Solid Edge part; units mm, degrees
sketch "Sketch1" plane through (0, 0, 0) normal (0, -1, 0) x (1, 0, 0)
  line L0 (12, 0) -> (12, 0.95)
  line L1 (12, 0.95) -> (1.25, 0.95)
  line L2 (1.25, 1.63) -> (1.25, 0.95)
  spline S0 degree 3 poles (0, 0) (0, 0.7831) (0.4356, 1.448) (1.25, 1.63) knots 0 0 0 0 1 1 1 1
revolve "RevolvedProtrusion1" add sketch "Sketch1" angle 360 about axis through (0, 0, 0) along (1, 0, 0)
sketch "Sketch2" plane through (0, 0, 0) normal (1, 0, 0) x (0, 0, 1)
  line L0 (-0.375, 1.9976) -> (0.375, 1.9976)
  line L1 (0.375, 1.9976) -> (0.375, 0.6495)
  arc A0 (0.375, 0.6495) -> (0.375, -0.6495) centre (0, 0) cw
  line L2 (0.375, -0.6495) -> (0.375, -1.9976)
  line L3 (0.375, -1.9976) -> (-0.375, -1.9976)
  line L4 (-0.375, -1.9976) -> (-0.375, -0.6495)
  line L5 (-0.375, 0.6495) -> (-0.375, 1.9976)
  arc A1 (-0.375, -0.6495) -> (-0.375, 0.6495) centre (0, 0) cw
extrude "Cutout1" cut sketch "Sketch2" along normal blind 0.6
fillet "Round_1" radius 0.15 2 edges at (12, 0, -0.95) (1.25, 0, -1.63)
properties material "Galvanized steel"
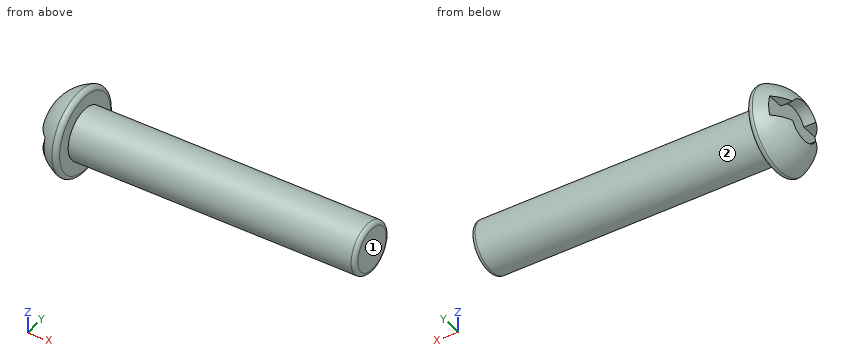
Work out the finished part from the listing and answer in its coordinate system (mm). Face numbers are marked on the shaded views. A direction names the side the tool comes from. Coordinates: 2 decimals unless noted, no trailing zeros. Order: outer loops, then holes, each group sorted by start corner. A loop starts at its lowest first (then second) coordinate and runs counter-clockwise, first axis right, second up. Notation, with made-up numbers: (14.5, 37.25) - (67.5, 37.25) arc R29 ccw to (67.5, 65.25) - close; hole circle Ø9 at (-27, 46.25). An arc over 180 degrees is marked (long way). Put each result on its own line as item: value. Start each with the question number.
1) Find the intervals of material crossed by line 1 (Z direction, x = 9.5, y = -0.05); line 2 (Z direction, x = 6.5, y = 0.65); line 3 (X direction, y = -0.55, z = 1.1), in increasing order. Write a range as from..to.
2) Flat-ended cylindrical pins translate along their axes: pin 1 (1.5 mm diameter, centred on x = 8.5, y = 0.5, fed in from -Z); pin 2 (0.5 mm diameter, centred on y = -0.5, z = 0, fed in from -X). Find the tip coordinate at first contact, or state that the pin passes through.
3) Find section A-A (x = 3). Give the vertices of the cut face in (y, z).
4) For the marked faces 1 and 2, determine the directions among +Z, -Z, +X, -X, +Y, -Y from which every point of the face is accessible in a straight line to the end or side of a thin tool.
Results list:
1. line 1: z = -0.95..0.95
1. line 2: z = -0.69..0.69
1. line 3: x = 0.49..1.25
2. pin 1: stops at z = -0.95
2. pin 2: stops at x = 0.6
3. outline: circle Ø1.9 at (0, 0)
4. face 1: +Z, -Z, +X, +Y, -Y
4. face 2: +X
